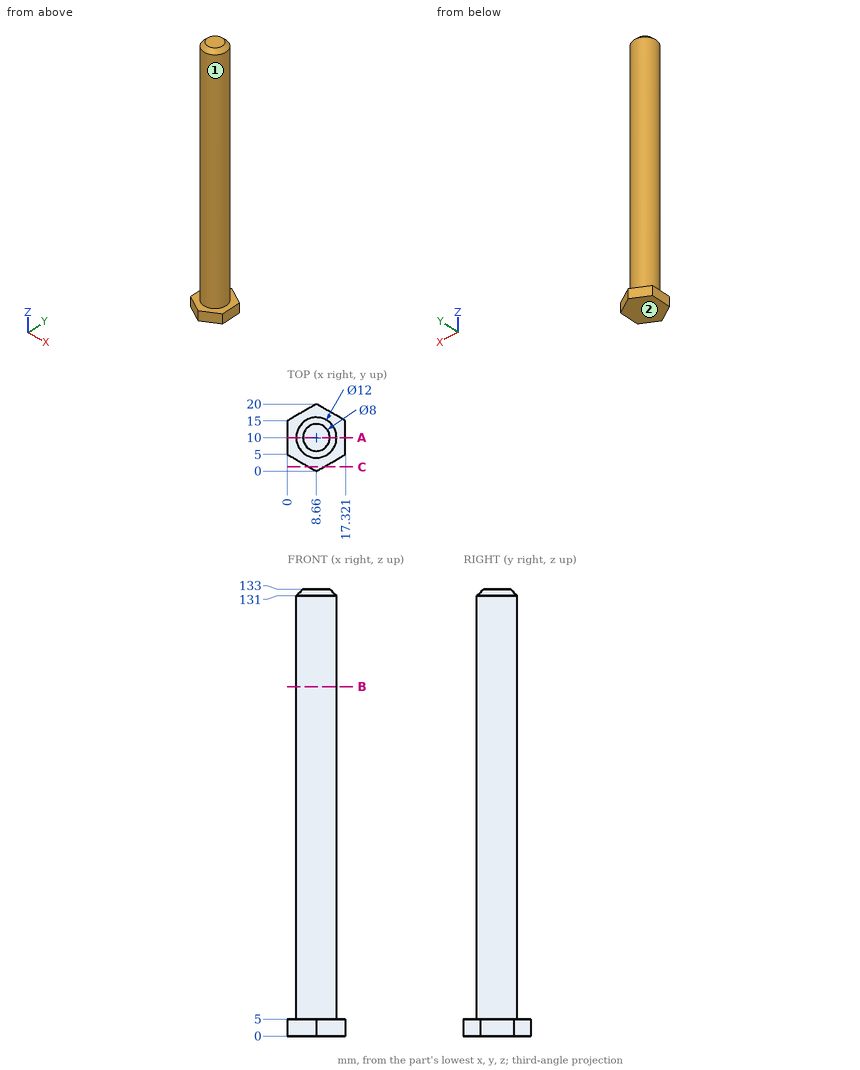
Design review of the part shown in the three views and the two pictorial views. Dimensions are in mm from the part's minimum x, y and z. A direction names the side the tool comes from. Coordinates: 2 decimals unless noted, no trailing zeros. Write each loop counter-clockwise with the first axis right and the second up, starting at its lowest first coordinate (ties: lowest second). Pieces come first, ordered by that corner, then holes. Notation, with made-up numbers: (10, -38.75) - (34, -38.75) arc R14 ccw to (34, -18.75) - close; hole circle Ø9 at (31.5, 19.5). An arc over 180 degrees is marked (long way). Write item = value, one per line.
(1) Consider section C-C, the plane y = 1.25. Give the boundary of the cut face in (x, z) (1 decimal).
Result sheet:
outline = (6.5, 0) - (10.8, 0) - (10.8, 5) - (6.5, 5) - close
(2) For P1, Ø6, axis at x = 11.5, z = 87, coming from the -Y side; P2, Ø5, axis at x = 12.5, z = 50.5, coming from the +Y side; P3, Ø4, axis at x = 14.5, y = 6.5, coming from the +Z side, all flat-tipped, find the tip position at first contact; note any pin that passes through.
Result sheet:
P1 = 4
P2 = 15.85
P3 = 132.19
(3) Consider section B-B, the plane z = 104. Give the boundary of the cut face in (x, y).
Result sheet:
outline = circle Ø12 at (8.66, 10)
(4) Consider section A-A, the plane y = 10. Give the boundary of the cut face in (x, z), then the cut area to 3 significant figures.
Result sheet:
outline = (0, 0) - (17.32, 0) - (17.32, 5) - (14.66, 5) - (14.66, 131) - (12.66, 133) - (4.66, 133) - (2.66, 131) - (2.66, 5) - (0, 5) - close
area = 1,620 mm^2
(5) Machinability: for the marked faces 1 and 2, which of the approach directions +Z, -Z, +X, -X, +Y, -Y give a long, thin tool a straight path to every point of the face, cutting with its end or side? Answer none if there is none.
Result sheet:
face_1 = +Z
face_2 = -Z, +X, -X, +Y, -Y
(6) For line 1 (Z direction, x = 2, y = 8.75); line 2 (Y direction, x = 8.5, z = 122); line 3 (Y direction, x = 5.5, z = 111.5), list the stretches that pass through material, from the lowest coordinate up. Write a range as [from, to].
Result sheet:
line_1 = [0, 5]
line_2 = [4, 16]
line_3 = [4.9, 15.1]
